The listing builds one solid part. Answer for the finished solid, in the listing's coordinates (mm). Face numbers are marked on the shaded views. A direction names the side the tool comes from. Coordinates: 2 decimals unless noted, no trailing zeros. Loops run counter-clockwise (first coordinate to the right, second up) from the corner with the lowest first, then second, coordinate; pieces in that order, holes last. Notation, with made-up numbers: (-25.75, -25) - (-13.75, -25) arc R16 ccw to (-13.75, -14) - close; hole circle Ø8 at (-12.75, 73). An arc over 180 degrees is marked (long way). Write each question's results on one line, items separated by ' | '. Start each with the question number.
(1) Find section B-B on x = -41.75. State how many separate pieces and enclosed holes the cut face has, then the cut area to 3 significant figures.
(2) For the marked faces 4 and 5, determine the directions among +Z, -Z, +X, -X, +Y, -Y from which every point of the face is accessible in a straight line to the end or side of a thin tool.
(3) Consider line 1 (Z direction, x = -28.25, y = 12.25); line 2 (Z direction, x = -41.75, y = 9); line 3 (X direction, y = 11.25, z = -22.5). Determine where each line is inside the solid, lowest interval first. Write a range as from..to.
(4) Find section D-D on z = -21.5. Determine the outline of the cut face in (x, y).
(5) Find section C-C on z = -26.5. Determine the outline of the cut face in (x, y), then the cut area to 3 significant figures.
(6) Given pin 1 Ø9 at (x, z) = (-21.5, -21.5) entering from -Y; pin 2 Ø3.5 at (x, z) = (-28.25, -9.81) entering from +Y; pin 3 Ø2 at (x, y) = (-42.5, 4) entering from -Z; pin 4 Ø2 at (x, y) = (-18.5, 7) entering from -Z, each flat-ended and moving along its own axis, determine where each tip first touches the part or whether it passes through.
(7) Determine the mould class of the marked faces 1, 2 and 3 for opening direction Z: released by +Z, released by -Z, zero draft, split by the parting line, or undercut.
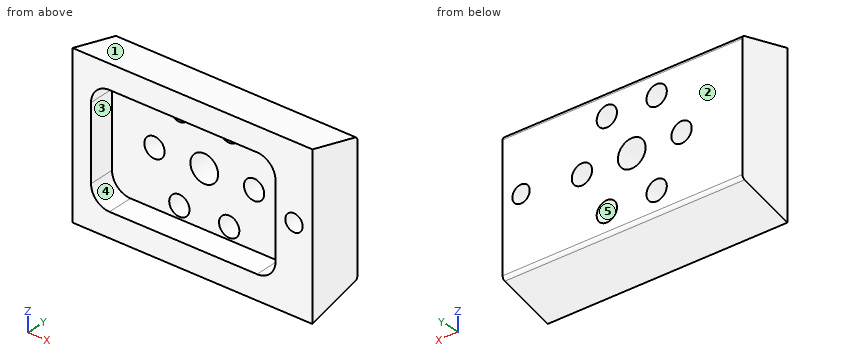
Autodesk Inventor part; units mm, degrees
ref_plane "YZ Plane" through (0, 0, 0) normal (1, 0, 0) x (0, 1, 0)
ref_plane "XZ Plane" through (0, 0, 0) normal (0, 1, 0) x (-1, 0, 0)
ref_plane "XY Plane" through (0, 0, 0) normal (0, 0, 1) x (1, 0, 0)
sketch "Sketch1" plane through (0, 0, 0) normal (0, 1, 0) x (-1, 0, 0)
  line L0 (0, 0) -> (65, 0)
  line L1 (65, 0) -> (65, -43)
  line L2 (65, -43) -> (0, -43)
  line L3 (0, -43) -> (0, 0)
  dimension "d0" = 65
  dimension "d1" = 43
extrude "Extrusion1" add sketch "Sketch1" along normal blind 15
sketch "Sketch2" plane through (0, 0, 0) normal (0, -1, 0) x (1, 0, 0)
  line L0 (-55, -36.5) -> (-15, -36.5)
  line L1 (-10, -31.5) -> (-10, -11.5)
  line L2 (-15, -6.5) -> (-55, -6.5)
  line L3 (-60, -11.5) -> (-60, -31.5)
  line L4 (-65, 0) -> (0, 0)
  line L5 (0, -43) -> (-65, -43)
  line L6 (0, 0) -> (0, -43)
  line L7 (-65, -43) -> (-65, 0)
  arc A0 (-10, -11.5) -> (-15, -6.5) centre (-15, -11.5) ccw
  arc A1 (-55, -6.5) -> (-60, -11.5) centre (-55, -11.5) ccw
  arc A2 (-60, -31.5) -> (-55, -36.5) centre (-55, -31.5) ccw
  arc A3 (-15, -36.5) -> (-10, -31.5) centre (-15, -31.5) ccw
  dimension "d4" = 6.5
  dimension "d5" = 6.5
  dimension "d6" = 10
  dimension "d7" = 5
  dimension "d8" = 5
extrude "Extrusion2" cut sketch "Sketch2" against normal blind 7 contours A2 L3 A1 L2 A0 L1 A3 L0
sketch "Sketch3" plane through (0, 7, 0) normal (0, -1, 0) x (1, 0, 0)
  circle A0 centre (-35, -21.5) radius 3.75
  line L0 (-10, -11.5) -> (-10, -31.5)
  line L1 (-15, -36.5) -> (-55, -36.5)
  point P0 (0, 0)
  dimension "d11" = 7.5
  dimension "d12" = 25
  dimension "d13" = 15
extrude "Extrusion3" cut sketch "Sketch3" against normal blind 8
thread "Thread1"
sketch "Sketch4" plane through (0, 0, 0) normal (0, -1, 0) x (1, 0, 0)
  circle A0 centre (-5, -20) radius 2.35
  line L0 (-65, 0) -> (0, 0)
  line L1 (0, 0) -> (0, -43)
  dimension "d18" = 4.7
  dimension "d19" = 20
  dimension "d20" = 5
extrude "Extrusion4" cut sketch "Sketch4" against normal blind 15
thread "Thread2"
chamfer "Chamfer1" distance 4 distance2 15 2 edges at (-32.5, 15, -43) (-32.5, 15, 0) measured on face at (-33.1827, 15, -37.0742)
fillet "Fillet1" radius 1 2 edges at (-32.5, 15, -39.0005) (-32.5, 15, -3.9995)
sketch "Sketch5" plane through (0, 15, 0) normal (0, 1, 0) x (1, 0, 0)
  circle A0 centre (-21.5, 21.5) radius 2.75
  circle A1 centre (-35, 21.5) radius 3.75
  circle A2 centre (-28.25, 33.1913) radius 2.75
  circle A3 centre (-41.75, 33.1913) radius 2.75
  circle A4 centre (-48.5, 21.5) radius 2.75
  circle A5 centre (-41.75, 9.8087) radius 2.75
  circle A6 centre (-28.25, 9.8087) radius 2.75
  point P0 (0, 0)
  dimension "d29" = 5.5
  dimension "d30" = 13.5
  dimension "d33" = 360
extrude "Extrusion5" cut sketch "Sketch5" against normal blind 15 contours A0 | A2 | A3 | A4 | A5 | A6
properties part number "Wedge-Dove tail"
Values:
1) separate pieces: 3 | enclosed holes: 0 | area: 287 mm²
2) face 4: -Y | face 5: +Y, -Y
3) line 1: z = -39.73..-35.94, -30.44..-12.56, -7.06..-3.27 | line 2: z = -40.6..-35.94, -30.44..-12.56, -7.06..-2.4 | line 3: x = -65..-51.06, -45.94..-38.61, -31.39..-24.06, -18.94..0
4) outline: (-65, 0) - (-60, 0) - (-60, 7) - (-51.25, 7) - (-51.25, 15) - (-65, 15) - close; (-45.75, 7) - (-38.75, 7) - (-38.75, 15) - (-45.75, 15) - close; (-31.25, 7) - (-24.25, 7) - (-24.25, 15) - (-31.25, 15) - close; (-18.75, 7) - (-10, 7) - (-10, 0) - (-6.81, 0) - (-6.81, 15) - (-18.75, 15) - close; (-3.19, 0) - (0, 0) - (0, 15) - (-3.19, 15) - close
5) outline: (-65, 0) - (-60, 0) - (-60, 7) - (-10, 7) - (-10, 0) - (0, 0) - (0, 15) - (-65, 15) - close | area: 625 mm²
6) pin 1: stops at y = 7 | pin 2: passes through | pin 3: stops at z = -42.2 | pin 4: stops at z = -41.4
7) face 1: released by +Z | face 2: zero draft | face 3: undercut
